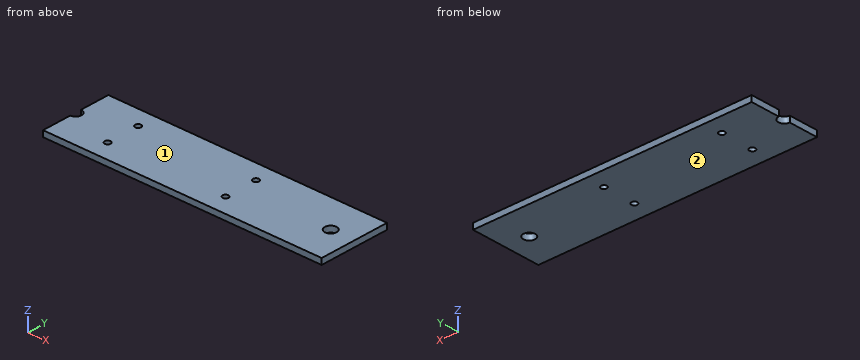
Autodesk Inventor part; units mm, degrees
ref_plane "YZ Plane" through (0, 0, 0) normal (1, 0, 0) x (0, 1, 0)
ref_plane "XZ Plane" through (0, 0, 0) normal (0, 1, 0) x (-1, 0, 0)
ref_plane "XY Plane" through (0, 0, 0) normal (0, 0, 1) x (1, 0, 0)
sketch "Sketch2" plane through (0, 0, 0) normal (0, 0, 1) x (1, 0, 0)
  line L0 (0, 0) -> (150.0124, 0)
  line L1 (150.0124, 0) -> (150.0124, 38.1)
  line L2 (150.0124, 38.1) -> (0, 38.1)
  line L3 (0, 38.1) -> (0, 0)
  circle A0 centre (137.3124, 19.05) radius 3.175
  circle A1 centre (25.4, 27.94) radius 1.5875
  circle A2 centre (88.9, 27.94) radius 1.5875
  circle A3 centre (88.9, 10.16) radius 1.5875
  circle A4 centre (25.4, 10.16) radius 1.5875
  circle A5 centre (0, 19.05) radius 3.175
  point P0 (0, 22.225)
  point P1 (0, 15.875)
  dimension "d0" = 150.0124
  dimension "d1" = 38.1
  dimension "d2" = 6.35
  dimension "d3" = 3.175
  dimension "d4" = 3.175
  dimension "d5" = 3.175
  dimension "d6" = 3.175
  dimension "d7" = 6.35
  dimension "d8" = 25.4
  dimension "d9" = 10.16
  dimension "d10" = 10.16
  dimension "d12" = 88.9
  dimension "d13" = 88.9
  dimension "d14" = 10.16
  dimension "d15" = 10.16
  dimension "d16" = 25.4
  dimension "d17" = 19.05
  dimension "d18" = 12.7
extrude "Extrusion1" add sketch "Sketch2" along normal blind 3.175 contours L3 A5 L2 L1 L0
properties part number "arm counterweight"
Verification items for the finished model (mm, model axes). Face numbers are marked on the shaded views. Coordinates: 2 decimals unless noted, no trailing zeros. Order: outer loops, then holes, each group sorted by start corner. A loop starts at its lowest first (then second) coordinate and runs counter-clockwise, first axis right, second up. Notation, with made-up numbers: M 34.25,65 L 77.25,65 A20 cw 77.25,97 Z; hole C 63,-1.75 d3. An arc over 180 degrees is marked long. One line per item, written item: value. Start each with the question number.
Item 1: Thickness scan on probe 1 along Y at (x, z) = (25.4, 0.7); probe 2 along X at (y, z) = (28, 1.3); probe 3 along X at (y, z) = (29, 1.9). Record the ranges inside material, lowest first.
Item 2: Sectioned sample at B-B on y = 27.94. Record the cut outline in (x, z) (1 decimal), then the cut area to 3 significant figures.
Item 3: Depth check by flat-ended pin: P1, Ø1.9, axis at x = 88.9, y = 27.94, coming from the -Z side; P2, Ø3.5, axis at x = 25.4, y = 10.16, coming from the -Z side. Enter the tip coordinate at first touch or a pass-through.
Item 4: Sectioned sample at A-A on x = 88.9. Record the cut outline in (y, z) (1 decimal), then the cut area to 3 significant figures.
Item 5: Mould release check, pull along Z, two halves, no side actions. Record for the marked faces 1 and 2: pulls with the +Z half, pulls with the -Z half, needs draft (parallel to the pull), parting line crosses it, or undercut.
Calculated:
1. probe 1: 0 to 8.57, 11.75 to 26.35, 29.53 to 38.1
1. probe 2: 0 to 23.81, 26.99 to 87.31, 90.49 to 150.01
1. probe 3: 0 to 24.22, 26.58 to 87.72, 90.08 to 150.01
2. outline: M 0,0 L 23.8,0 L 23.8,3.2 L 0,3.2 Z; M 27,0 L 87.3,0 L 87.3,3.2 L 27,3.2 Z; M 90.5,0 L 150,0 L 150,3.2 L 90.5,3.2 Z
2. area: 456 mm^2
3. P1: through
3. P2: z = 0
4. outline: M 0,0 L 8.6,0 L 8.6,3.2 L 0,3.2 Z; M 11.7,0 L 26.4,0 L 26.4,3.2 L 11.7,3.2 Z; M 29.5,0 L 38.1,0 L 38.1,3.2 L 29.5,3.2 Z
4. area: 101 mm^2
5. face 1: pulls with the +Z half
5. face 2: pulls with the -Z half
